```python
from build123d import *

# Parameters (mm, degrees)
EXTRUDE_1_DEPTH     = 20
SKETCH_2_R          = 1.85
CUT_EXTRUDE_1_DEPTH = 6
SKETCH_3_R          = 1.125
CUT_EXTRUDE_2_DEPTH = 20.825317547
SKETCH_4_OUTSIDE_W  = 36.206
SKETCH_4_OUTSIDE_H  = 39.867
CUT_EXTRUDE_3_DEPTH = 21
SKETCH_5_W          = 4
SKETCH_5_H          = 15
SKETCH_5_H_2        = 0.9
CUT_EXTRUDE_4_DEPTH = 21
SKETCH_6_W          = 4
SKETCH_6_H          = 7
CUT_EXTRUDE_5_DEPTH = 6.207259422
SKETCH_7_W          = 8
SKETCH_7_H          = 0.5
CUT_EXTRUDE_6_DEPTH = 21
CUT_EXTRUDE_7_DEPTH = 2


with BuildPart() as part:
    # Эскиз1 → Бобышка-Вытянуть1 (new body)
    with BuildSketch(Plane.XY):
        Polygon((-12.5, 21.650635095), (0, 0), (12.990381057, 7.5), (0.490381057, 29.150635095), align=None)
    extrude(amount=EXTRUDE_1_DEPTH)

    # Эскиз2 → Вырез-Вытянуть1 (cut)
    with BuildSketch(Plane(origin=(12.990381057, 7.5, 0), x_dir=(0, 0, -1), z_dir=(0.866025404, 0.5, 0))):
        with Locations((-10, 8)):
            Circle(SKETCH_2_R)
    extrude(amount=-CUT_EXTRUDE_1_DEPTH, mode=Mode.SUBTRACT)

    # Эскиз3 → Вырез-Вытянуть2 (cut, through all)
    with BuildSketch(Plane(origin=(7.794228634, 4.5, 0), x_dir=(0, 0, -1), z_dir=(0.866025404, 0.5, 0))):
        with Locations((-10, 8)):
            Circle(SKETCH_3_R)
    extrude(amount=-CUT_EXTRUDE_2_DEPTH, mode=Mode.SUBTRACT)

    # Эскиз4 outside → Вырез-Вытянуть3 (cut, through all)
    with BuildSketch(Plane.XY.offset(20)):
        with Locations((0.245, 14.5755)):
            Rectangle(SKETCH_4_OUTSIDE_W, SKETCH_4_OUTSIDE_H)
        Polygon((-3.75, 6.495190528), (11.25, 6.495190528), (11.25, 10.514428415), (1.903841409, 26.70244995), (-3.75, 26.70244995), align=None, mode=Mode.SUBTRACT)
    extrude(amount=-CUT_EXTRUDE_3_DEPTH, mode=Mode.SUBTRACT)

    # Эскиз5 → Вырез-Вытянуть4 (cut, through all)
    with BuildSketch(Plane.XY.offset(20)):
        with Locations((-1.75, 19.20244995)):
            Rectangle(SKETCH_5_W, SKETCH_5_H)
        with Locations((-1.75, 6.945190528)):
            Rectangle(SKETCH_5_W, SKETCH_5_H_2)
    extrude(amount=-CUT_EXTRUDE_4_DEPTH, mode=Mode.SUBTRACT)

    # Эскиз6 → Вырез-Вытянуть5 (cut, through all)
    with BuildSketch(Plane(origin=(0, 11.70244995, 0), x_dir=(1, 0, 0), z_dir=(0, 1, 0))):
        with Locations((-1.75, -16.5)):
            Rectangle(SKETCH_6_W, SKETCH_6_H)
        with Locations((-1.75, -3.5)):
            Rectangle(SKETCH_6_W, SKETCH_6_H)
    extrude(amount=-CUT_EXTRUDE_5_DEPTH, mode=Mode.SUBTRACT)

    # Эскиз7 → Вырез-Вытянуть6 (cut, through all)
    with BuildSketch(Plane.XY.offset(20)):
        Polygon((0.25, 21.022474586), (5.183176715, 21.022474586), (1.903841409, 26.70244995), (0.25, 26.70244995), align=None)
        with Locations((4.25, 6.745190528)):
            Rectangle(SKETCH_7_W, SKETCH_7_H)
    extrude(amount=-CUT_EXTRUDE_6_DEPTH, mode=Mode.SUBTRACT)

    # Эскиз8 → Вырез-Вытянуть7 (cut)
    with BuildSketch(Plane.XZ.offset(-6.995190528)):
        with BuildLine():
            Line((-3.75, 11.505998369), (0.25, 11.505998369))
            ThreePointArc((0.25, 11.505998369), (1.755998369, 10), (0.25, 8.494001631))
            Line((0.25, 8.494001631), (-3.75, 8.494001631))
            Line((-3.75, 8.494001631), (-3.75, 11.505998369))
        make_face()
    extrude(amount=-CUT_EXTRUDE_7_DEPTH, mode=Mode.SUBTRACT)


solid = part.part
```
For this review, take the finished solid that the model builds, in its own axes (mm). A direction names the side the tool comes from. Round coordinates to 2 decimals unless told otherwise and drop trailing zeros. Write each loop counter-clockwise with the first axis right and the second up, starting at its lowest first coordinate (ties: lowest second). Pieces come first, ordered by that corner, then holes. Notation, with made-up numbers: (-28.75, -21.5) - (7.25, -21.5) arc R24 ccw to (7.25, -10.5) - close; hole circle Ø3 at (35, 10.25). An arc over 180 degrees is marked (long way). Put each result on its own line as item: value.
Q1. Wall thickness on probe 1 along Y at (x, z) = (2, 1); probe 2 along X at (y, z) = (14.5, 6.25); probe 3 along Y at (x, z) = (1.25, 9.5): over which ranges is each line inside the solid? List them lowest first.
Solved:
probe 1: y = 7 to 21.02
probe 2: x = 0.25 to 8.95
probe 3: y = 11.12 to 21.02
Q2. Machinability: for faces 1 (the face through (-2, 10, 13)), 2 (the face through (-2, 8, 8.494)), 3 (the face through (-2, 10, 7)), 4 (the face through (4, 6.995, 10)), which of the approach directions +Z, -Z, +X, -X, +Y, -Y give a long, thin tool a straight path to every point of the face, cutting with its end or side? Answer none if there is none.
Solved:
face 1: +Z, -X, +Y, -Y
face 2: -X, -Y
face 3: -Z, -X, +Y, -Y
face 4: +Z, -Z, -X, -Y
Q3. We need section B-B (z = 10). Give the boundary of the cut face in (x, y).
Solved:
outline: (-3.75, 9) - (-2.67, 9) - (3.23, 12.4) - (2.87, 13.03) - (8.07, 16.03) - (5.18, 21.02) - (0.25, 21.02) - (0.25, 11.7) - (-3.75, 11.7) - close; (1.76, 7) - (8.25, 7) - (8.25, 6.5) - (11.25, 6.5) - (11.25, 10.51) - (9.92, 12.83) - (4.72, 9.83) - (4.36, 10.45) - (1.76, 8.95) - close
Q4. We need section A-A (y = 8). Give the boundary of the cut face in (x, z).
Solved:
outline: (-3.75, 7) - (0.25, 7) - (0.25, 0) - (11.25, 0) - (11.25, 20) - (0.25, 20) - (0.25, 13) - (-3.75, 13) - (-3.75, 11.51) - (0.25, 11.51) arc R1.51 cw to (0.25, 8.49) - (-3.75, 8.49) - close
Q5. Mouldability with a two-part tool opening along Y and no side actions: class faces 5 (the face through (10, 6.495, 10)), 6 (the face through (0.98, 11.09, 10.15)), 7 (the face through (11.25, 8, 10)) as released by +Y, released by -Y, zero draft, split by the parting line, or undercut.
Solved:
face 5: released by -Y
face 6: undercut
face 7: zero draft
Q6. We need section D-D (y = 18.75). Give the boundary of the cut face in (x, z), and give its area (3 significant figures).
Solved:
outline: (0.25, 0) - (6.5, 0) - (6.5, 20) - (0.25, 20) - close
area: 125 mm2
Q7. We need section C-C (z = 2.5). Give the boundary of the cut face in (x, y).
Solved:
outline: (0.25, 7) - (8.25, 7) - (8.25, 6.5) - (11.25, 6.5) - (11.25, 10.51) - (5.18, 21.02) - (0.25, 21.02) - close
Q8. Insertion check: pin 1 Ø3 at (x, y) = (-2, 10.5) entering from +Z; pin 2 Ø0.7 at (x, z) = (-2.5, 12.5) entering from -Y; pin 3 Ø2.5 at (x, z) = (-2, 10) entering from -Y. Each pin has a flat end and moves straight along its axis. Give the tip position at first contact, or say it passes through.
Solved:
pin 1: stops at z = 13
pin 2: stops at y = 7.4
pin 3: stops at y = 9
